Can you work these out from the drawing? Everything is in mm from the part's minimum corner. A direction names the side the tool comes from. Round coordinates to 2 decimals unless told otherwise and drop trailing zeros. Order: outer loops, then holes, each group sorted by start corner. A loop starts at its lowest first (then second) coordinate and runs counter-clockwise, first axis right, second up. Notation, with made-up numbers: (-8, 38.25) - (7, 38.25) arc R20 ccw to (7, 51.25) - close; hole circle Ø6 at (59, 78). An arc over 180 degrees is marked (long way). Answer as a JSON object with one key per item and string values.
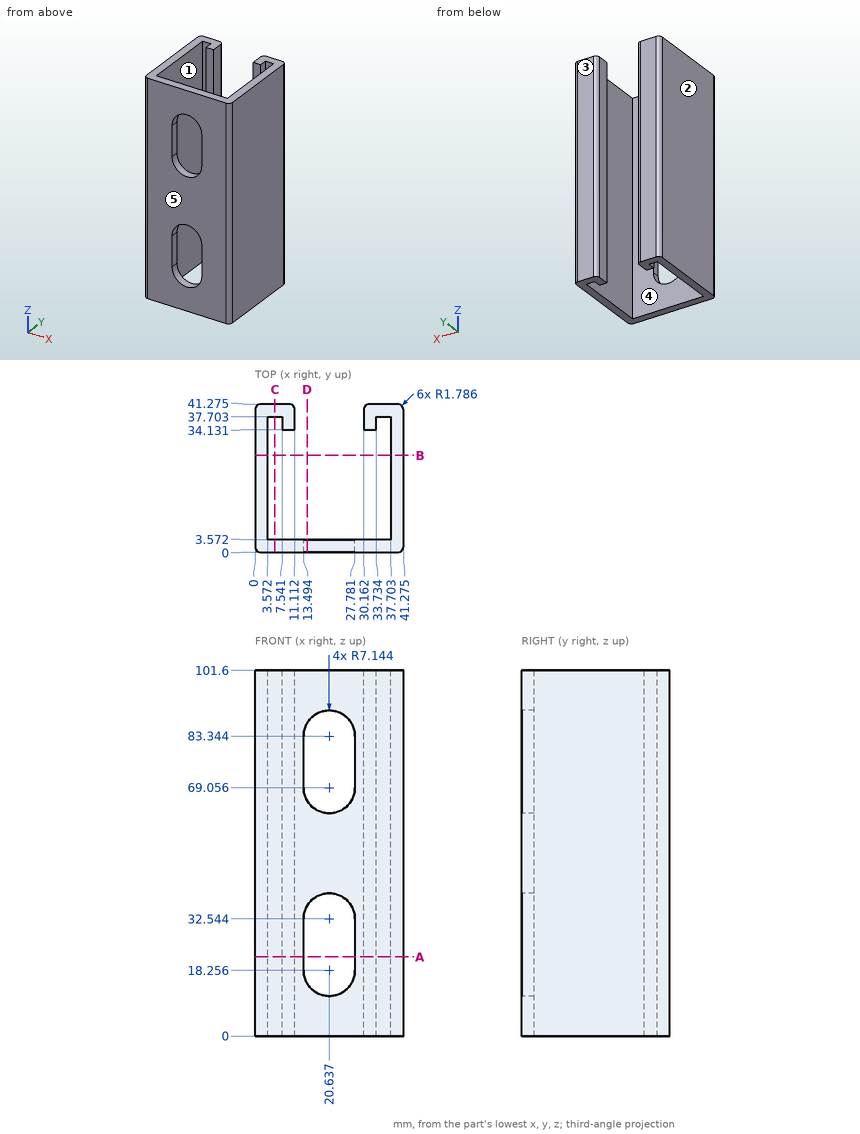
1. For P1, Ø10, axis at x = 24, z = 59, coming from the +Y side, with a flat end and sliding along its axis, tell me the tip position at first contact or that it passes through.
Responses:
{"P1": "y = 3.57"}
2. If I drill on L1, parallel to X at y = 35.5, z = 27.5 (1 decimal); L2, parallel to X at y = 19.5, z = 80 (1 decimal); L3, parallel to Y at x = 32, z = 10.5 (1 decimal), over which ranges is the centre line in solid material (lowest first)? Write a range as [from, to].
Responses:
{"L1": "[0, 3.6], [7.5, 11.1], [30.2, 33.7], [37.7, 41.3]", "L2": "[0, 3.6], [37.7, 41.3]", "L3": "[0, 3.6], [34.1, 41.3]"}
3. Imagine slicing it at B-B (y = 27). List the corners of the cut face in (x, z) for me (1 decimal).
Responses:
{"outline": "(0, 0) - (3.6, 0) - (3.6, 101.6) - (0, 101.6) - close; (37.7, 0) - (41.3, 0) - (41.3, 101.6) - (37.7, 101.6) - close"}
4. Imagine slicing it at A-A (z = 22). List the corners of the cut face in (x, y) for me (1 decimal).
Responses:
{"outline": "(0, 1.8) arc R1.8 ccw to (1.8, 0) - (13.5, 0) - (13.5, 3.6) - (3.6, 3.6) - (3.6, 37.7) - (7.5, 37.7) - (7.5, 34.1) - (11.1, 34.1) - (11.1, 39.5) arc R1.8 ccw to (9.3, 41.3) - (1.8, 41.3) arc R1.8 ccw to (0, 39.5) - close; (27.8, 0) - (39.5, 0) arc R1.8 ccw to (41.3, 1.8) - (41.3, 39.5) arc R1.8 ccw to (39.5, 41.3) - (31.9, 41.3) arc R1.8 ccw to (30.2, 39.5) - (30.2, 34.1) - (33.7, 34.1) - (33.7, 37.7) - (37.7, 37.7) - (37.7, 3.6) - (27.8, 3.6) - close"}
5. For the marked faces 4 and 5, which set-ups out of +Z, -Z, +X, -X, +Y, -Y let a thin tool reach every point of the face, with its end or its side?
Responses:
{"face 4": "+Z, -Z", "face 5": "+Z, -Z, +X, -X, -Y"}
6. Thinking about a two-plate mould opening in X: for the marked faces 1, 2 and 3, which applies, pulls with the +X half, pulls with the -X half, needs draft (parallel to the pull), parting line crosses it, or undercut?
Responses:
{"face 1": "undercut", "face 2": "pulls with the -X half", "face 3": "needs draft"}
7. Imagine slicing it at D-D (x = 14.5). List the corners of the cut face in (y, z) for me.
Responses:
{"outline": "(0, 0) - (3.57, 0) - (3.57, 14.6) - (0, 14.6) - close; (0, 36.2) - (3.57, 36.2) - (3.57, 65.4) - (0, 65.4) - close; (0, 87) - (3.57, 87) - (3.57, 101.6) - (0, 101.6) - close"}
